```python
from build123d import *

# Parameters (mm, degrees)
SKETCH1_W           = 100
SKETCH1_H           = 200.1518
BOSS_EXTRUDE1_DEPTH = 6.35
SKETCH2_W           = 6.35
SKETCH2_H           = 50.8
SKETCH2_H_2         = 49.2759
CUT_EXTRUDE1_DEPTH  = 6.35
SKETCH3_W           = 61.9
SKETCH3_H           = 174.7518
CUT_EXTRUDE2_DEPTH  = 6.35
FILLET1_R           = 12.7
SKETCH6_W           = 6.35
SKETCH6_H           = 6.35
BOSS_EXTRUDE2_DEPTH = 2.54
SKETCH7_W           = 6.35
SKETCH7_H           = 6.35
BOSS_EXTRUDE3_DEPTH = 2.54


with BuildPart() as part:
    # Sketch1 → Boss-Extrude1 (new body)
    with BuildSketch(Plane.XY):
        with Locations((0, -50.0759)):
            Rectangle(SKETCH1_W, SKETCH1_H)
    extrude(amount=BOSS_EXTRUDE1_DEPTH)

    # Sketch2 → Cut-Extrude1 (cut)
    with BuildSketch(Plane.XY.offset(6.35)):
        with Locations((-46.825, -24.6759)):
            Rectangle(SKETCH2_W, SKETCH2_H)
        with Locations((-46.825, -75.4759)):
            Rectangle(SKETCH2_W, SKETCH2_H)
        with Locations((46.825, 25.36205)):
            Rectangle(SKETCH2_W, SKETCH2_H_2)
        with Locations((46.825, -125.51385)):
            Rectangle(SKETCH2_W, SKETCH2_H_2)
    extrude(amount=-CUT_EXTRUDE1_DEPTH, mode=Mode.SUBTRACT)

    # Sketch3 → Cut-Extrude2 (cut)
    with BuildSketch(Plane.XY.offset(6.35)):
        with Locations((0, -50.0759)):
            Rectangle(SKETCH3_W, SKETCH3_H)
    extrude(amount=-CUT_EXTRUDE2_DEPTH, mode=Mode.SUBTRACT)

    # Fillet1
    fillet1_edges = [part.edges().sort_by_distance(p)[0] for p in [
        (-30.95, -137.4518, 3.175),
        (-30.95, 37.3, 3.175),
        (30.95, 37.3, 3.175),
        (30.95, -137.4518, 3.175),
    ]]
    fillet(fillet1_edges, radius=FILLET1_R)

    # Sketch6 → Boss-Extrude2 (add)
    with BuildSketch(Plane(origin=(0, 0.7241, 0), x_dir=(1, 0, 0), z_dir=(0, 1, 0))):
        with Locations((46.825, -3.175)):
            Rectangle(SKETCH6_W, SKETCH6_H)
    extrude(amount=BOSS_EXTRUDE2_DEPTH)

    # Sketch7 → Boss-Extrude3 (add)
    with BuildSketch(Plane.XZ.offset(100.8759)):
        with Locations((46.825, 3.175)):
            Rectangle(SKETCH7_W, SKETCH7_H)
    extrude(amount=BOSS_EXTRUDE3_DEPTH)


solid = part.part
```
Could you check a few things on this model? Use its own coordinates, in mm. A direction names the side the tool comes from. Coordinates: 2 decimals unless noted, no trailing zeros. Write each loop counter-clockwise with the first axis right and the second up, starting at its lowest first coordinate (ties: lowest second). Pieces come first, ordered by that corner, then holes. Notation, with made-up numbers: (-23.5, 29.5) -> (31.5, 29.5) arc R27 ccw to (31.5, 50.5) -> close; hole circle Ø4 at (61, 14). An arc over 180 degrees is marked (long way). Write item = value, one per line. Start each with the question number.
(1) Will these pins go through, and if not, where does the flat tip stop? pin 1 (1.9 mm diameter, centred on y = -32.5, z = 2.5, fed in from -X); pin 2 (1.9 mm diameter, centred on y = -136.5, z = 4.5, fed in from +X).
(2) I want a section at A-A (y = -11.5). Please give me the cut outline in (x, z), plus the area to 3 significant figures.
(3) I need wall thicknesses on line 1 (X direction, y = -44.5, z = 0.75); line 2 (Y direction, x = 2, z = 0.5); line 3 (X direction, y = -109, z = 4.5). Which ranges of each line are inside material? Lowest first, please. Write a range as [from, to].
(4) I want a section at B-B (x = 13.5). Please give me the cut outline in (y, z).
(5) We'd pull the mould along Y, two halves only. Please class faces 6 (the face through (-50, -126, 3)), 7 (the face through (-4, -150.152, 3)), 8 (the face through (27.33, 33.48, 3.13)): released by +Y, released by -Y, zero draft, split by the parting line, or undercut.
(6) I want a section at C-C (z = 2). Please give me the cut outline in (x, y).
(7) Which directions (+Z, -Z, +X, -X, +Y, -Y) give clear straight access to the entire face, cutting with the end or side of a thin tool? Please do faces 1 (the face through (33, -49, 0)), 2 (the face through (43.65, -127, 3)), 3 (the face through (-47, -100.876, 3)), 4 (the face through (50, -49, 3)), 5 (the face through (0, -137.452, 3)).
Result set:
q1.pin_1 = -43.65
q1.pin_2 = 43.65
q2.outline = (-43.65, 0) -> (-30.95, 0) -> (-30.95, 6.35) -> (-43.65, 6.35) -> close; (30.95, 0) -> (50, 0) -> (50, 6.35) -> (30.95, 6.35) -> close
q2.area = 202 mm2
q3.line_1 = [-43.65, -30.95], [30.95, 50]
q3.line_2 = [-150.15, -137.45], [37.3, 50]
q3.line_3 = [-50, -30.95], [30.95, 43.65]
q4.outline = (-150.15, 0) -> (-137.45, 0) -> (-137.45, 6.35) -> (-150.15, 6.35) -> close; (37.3, 0) -> (50, 0) -> (50, 6.35) -> (37.3, 6.35) -> close
q5.face_6 = zero draft
q5.face_7 = released by -Y
q5.face_8 = undercut
q6.outline = (-50, -150.15) -> (43.65, -150.15) -> (43.65, -103.42) -> (50, -103.42) -> (50, 3.26) -> (43.65, 3.26) -> (43.65, 50) -> (-50, 50) -> (-50, 0.72) -> (-43.65, 0.72) -> (-43.65, -100.88) -> (-50, -100.88) -> close; hole (-30.95, -124.75) arc R12.7 ccw to (-18.25, -137.45) -> (18.25, -137.45) arc R12.7 ccw to (30.95, -124.75) -> (30.95, 24.6) arc R12.7 ccw to (18.25, 37.3) -> (-18.25, 37.3) arc R12.7 ccw to (-30.95, 24.6) -> close
q7.face_1 = -Z, +X, -X, +Y, -Y
q7.face_2 = +Z, -Z, +X, -Y
q7.face_3 = +Z, -Z, -X
q7.face_4 = +Z, -Z, +X, +Y, -Y
q7.face_5 = +Z, -Z
